The model under review builds one solid part; all positions refer to its coordinate system, in mm. A direction names the side the tool comes from. Give positions to 0.01 mm unless a question says otherwise; leave off trailing zeros. Loops run counter-clockwise (first coordinate to the right, second up) from the corner with the lowest first, then second, coordinate; pieces in that order, holes last. Notation, with made-up numbers: (30.25, 9.25) - (37.25, 9.25) arc R20 cw to (37.25, 21.25) - close; hole circle Ø10 at (61, 57.25). An arc over 180 degrees is marked (long way). Return JSON: item names as keys, results as strings. Group by question number.
from build123d import *

# Parameters (mm, degrees)
SKETCH1_R               = 35
BOSS_EXTRUDE1_DEPTH     = 9
SKETCH2_R               = 2
CUT_EXTRUDE1_DEPTH      = 1
CUT_EXTRUDE1_DEPTH_BACK = 10
SKETCH3_R               = 29
SKETCH3_R_2             = 7
CUT_EXTRUDE2_DEPTH      = 7
SKETCH4_R               = 6
CUT_EXTRUDE3_DEPTH      = 3


with BuildPart() as part:
    # Sketch1 → Boss-Extrude1 (new body)
    with BuildSketch(Plane.XY):
        Circle(SKETCH1_R)
    extrude(amount=BOSS_EXTRUDE1_DEPTH)

    # Sketch2 → Cut-Extrude1 (cut, two sides)
    with BuildSketch(Plane.XY.offset(9)) as cut_extrude1_sk:
        Circle(SKETCH2_R)
    extrude(amount=CUT_EXTRUDE1_DEPTH, mode=Mode.SUBTRACT)
    extrude(cut_extrude1_sk.sketch, amount=-CUT_EXTRUDE1_DEPTH_BACK, mode=Mode.SUBTRACT)

    # Sketch3 → Cut-Extrude2 (cut)
    with BuildSketch(Plane.XY.offset(9)):
        Circle(SKETCH3_R)
        Circle(SKETCH3_R_2, mode=Mode.SUBTRACT)
    extrude(amount=-CUT_EXTRUDE2_DEPTH, mode=Mode.SUBTRACT)

    # Sketch4 → Cut-Extrude3 (cut, through all)
    with BuildSketch(Plane.XY.offset(2)):
        with Locations((0, 18)):
            Circle(SKETCH4_R)
        with Locations((15.588457268, 9)):
            Circle(SKETCH4_R)
        with Locations((15.588457268, -9)):
            Circle(SKETCH4_R)
        with Locations((0, -18)):
            Circle(SKETCH4_R)
        with Locations((-15.588457268, -9)):
            Circle(SKETCH4_R)
        with Locations((-15.588457268, 9)):
            Circle(SKETCH4_R)
    extrude(amount=-CUT_EXTRUDE3_DEPTH, mode=Mode.SUBTRACT)


solid = part.part
Item 1: Take a section at B-B (y = -23). State the section outline as (x, z) points.
Item 2: Take a section at D-D (z = 7.75). State the section outline as (x, y) points, then the cut area to 3 significant figures.
Item 3: Take a section at A-A (x = 0). State the section outline as (y, z) points.
Item 4: For P1, Ø9.5, axis at x = 0, y = -18, coming from the -Z side; P2, Ø17.5, axis at x = 13, y = 14.5, coming from the +Z side; P3, Ø1, axis at x = -13, z = 4.5, coming from the -Y side; P4, Ø1.5, axis at y = 22, z = 6.5, coming from the +X side, all flat-tipped, find the tip position at first contact; note any pin that passes through.
Item 5: Tool access review of faces 1 (the face through (-0.78, -12.05, 1.01)), 2 (the face through (6, -6, 2)): name each direction out of +Z, -Z, +X, -X, +Y, -Y from which nothing blocks a thin tool from reaching the whole face with its end or side.
Item 6: For L1, parallel to Y at x = 0, z = 1.5; L2, parallel to Y at x = 0, z = 3.75; L3, parallel to Y at x = 16, z = 1, list the stretches that pass through material, from the lowest coordinate up. Write a range as from..to.
Item 7: Take a section at C-C (z = 1). State the section outline as (x, y) points, then the cut area to 3 significant figures.
Item 8: Mouldability with a two-part tool opening along Y and no side actions: class faces 3 (the face through (-28, -21, 4)), 4 (the face through (13.38, -25.73, 5.55)), 5 (the face through (1, 2, 9)) as +Y half, -Y half, draft (parallel to the pull), parting line (faces both ways), or undercut.
Check sheet entries:
{
 "1": {"outline": "(-26.38, 0) - (-3.32, 0) - (-3.32, 2) - (-17.66, 2) - (-17.66, 9) - (-26.38, 9) - close; (3.32, 0) - (26.38, 0) - (26.38, 9) - (17.66, 9) - (17.66, 2) - (3.32, 2) - close"},
 "2": {"outline": "circle Ø70 at (0, 0); circle Ø14 at (0, 0); hole circle Ø58 at (0, 0); hole circle Ø4 at (0, 0)", "area": "1,350 mm^2"},
 "3": {"outline": "(-35, 0) - (-24, 0) - (-24, 2) - (-29, 2) - (-29, 9) - (-35, 9) - close; (-12, 0) - (-2, 0) - (-2, 9) - (-7, 9) - (-7, 2) - (-12, 2) - close; (2, 0) - (12, 0) - (12, 2) - (7, 2) - (7, 9) - (2, 9) - close; (24, 0) - (35, 0) - (35, 9) - (29, 9) - (29, 2) - (24, 2) - close"},
 "4": {"P1": "passes through", "P2": "stops at z = 2", "P3": "stops at y = -32.69", "P4": "stops at x = 27.81"},
 "5": {"face 1": "+Z, -Z", "face 2": "+Z"},
 "6": {"L1": "y = -35..-24, -12..-2, 2..12, 24..35", "L2": "y = -35..-29, -7..-2, 2..7, 29..35", "L3": "y = -31.13..-14.99, -3.01..3.01, 14.99..31.13"},
 "7": {"outline": "circle Ø70 at (0, 0); hole circle Ø12 at (-15.59, -9); hole circle Ø12 at (-15.59, 9); hole circle Ø12 at (0, -18); hole circle Ø12 at (0, 18); hole circle Ø4 at (0, 0); hole circle Ø12 at (15.59, -9); hole circle Ø12 at (15.59, 9)", "area": "3,160 mm^2"},
 "8": {"face 3": "parting line", "face 4": "undercut", "face 5": "draft"}
}
